Can you work these out from the model? Positions are in its coordinate system, mm. A direction names the side the tool comes from. Give positions to 0.01 mm unless a question says otherwise; leave off trailing zeros. Order: outer loops, then holes, each group sorted by start corner. A loop starts at its lowest first (then second) coordinate and runs counter-clockwise, first axis right, second up. Notation, with made-up numbers: (51, 50.5) -> (91, 50.5) arc R25 ccw to (91, 88.5) -> close; hole circle Ø10 at (-10, 45.5). An arc over 180 degrees is marked (long way). Answer as CSV lines item,"result".
```python
from build123d import *

# Parameters (mm, degrees)
F1_DEPTH = 0.635
F4_DEPTH = 25.4
F2_R     = 3.048
F6_DEPTH = 6.35
F7_DEPTH = 6.35


with BuildPart() as f1:
    # F0 (on Top) → F1 (new body)
    with BuildSketch(Plane.XY):
        with BuildLine():
            Line((0, 0), (89.802561, -89.802561))
            ThreePointArc((89.802561, -89.802561), (127, 0), (89.802561, 89.802561))
            Line((89.802561, 89.802561), (0, 0))
        make_face()
    extrude(amount=F1_DEPTH)

    # F3 (on face) → F4 (intersect)
    with BuildSketch(Plane.XY.offset(0.635)):
        with BuildLine():
            ThreePointArc((53.881537, 53.881537), (76.2, 0), (53.881537, -53.881537))
            Line((53.881537, -53.881537), (89.802561, -89.802561))
            ThreePointArc((89.802561, -89.802561), (127, 0), (89.802561, 89.802561))
            Line((89.802561, 89.802561), (53.881537, 53.881537))
        make_face()
    extrude(amount=-F4_DEPTH, mode=Mode.INTERSECT)

    # F2 (on face) → F6 (join)
    with BuildSketch(Plane.XY.offset(0.635)):
        with Locations((120.65, 0)):
            Circle(F2_R)
    extrude(amount=F6_DEPTH)

    # F5 (on face) → F7 (join)
    with BuildSketch(Plane.XY.offset(0.635)):
        with BuildLine():
            Line((75.810533, -18.372254), (75.810533, -37.168254))
            ThreePointArc((75.810533, -37.168254), (85.208533, -27.770254), (75.810533, -18.372254))
        make_face()
    extrude(amount=F7_DEPTH)


solid = f1.part
```
Item 1: Imagine slicing it at B-B, the plane y = 0. Please give me the cut outline in (x, z) (3 decimals), then the cut area to 3 significant figures.
Numbers:
outline,"(76.2, 0) -> (127, 0) -> (127, 0.635) -> (123.698, 0.635) -> (123.698, 6.985) -> (117.602, 6.985) -> (117.602, 0.635) -> (76.2, 0.635) -> close"
area,"71.0 mm²"
Item 2: Please list where these lines run through material, in increasing order: line 1 along Z through (x, y) = (117, 27.5) (3 decimals); line 2 along X through (y, z) = (-27.5, 3); line 3 along Y through (x, z) = (122, 5.5).
Numbers:
line 1,"z = 0 to 0.635"
line 2,"x = 75.81 to 85.2"
line 3,"y = -2.73 to 2.73"
Item 3: For faces 5 (the cylindrical face through (123.557, 0.916, 3.766)), 6 (the flat face through (72.1, 72.1, 0.3)), 7 (the flat face through (75.811, -28, 4)), which set-ups out of +Z, -Z, +X, -X, +Y, -Y let a thin tool reach every point of the face, with its end or its side?
Numbers:
face 5,"+Z"
face 6,"+Z, -Z, -X, +Y"
face 7,"+Z, -X, +Y, -Y"
Item 4: We'd pull the mould along Y, two halves only. Please class faces 1 (the cylindrical face through (76.195, 0.838, 0.322)), 2 (the flat face through (71.6, -71.6, 0.3)), 3 (the flat face through (90, 1, 0.635)), 4 (the cylindrical face through (85.206, -27.977, 3.766)): released by +Y, released by -Y, zero draft, split by the parting line, or undercut.
Numbers:
face 1,"undercut"
face 2,"released by -Y"
face 3,"zero draft"
face 4,"split by the parting line"
Item 5: Imagine slicing it at A-A, the plane z = 4.75. Please give me the cut outline in (x, y), then the cut area to 3 significant figures.
Numbers:
outline,"(75.81, -37.17) arc R9.4 ccw to (75.81, -18.37) -> close; circle Ø6.1 at (120.65, 0)"
area,"168 mm²"
Item 6: Imagine slicing it at D-D, the plane x = 106. Please give me the cut outline in (y, z) (3 decimals).
Numbers:
outline,"(-69.95, 0) -> (69.95, 0) -> (69.95, 0.635) -> (-69.95, 0.635) -> close"
Item 7: Imagine slicing it at C-C, the plane x = 120.65. Please give me the cut outline in (y, z) (3 decimals).
Numbers:
outline,"(-39.656, 0) -> (39.656, 0) -> (39.656, 0.635) -> (3.048, 0.635) -> (3.048, 6.985) -> (-3.048, 6.985) -> (-3.048, 0.635) -> (-39.656, 0.635) -> close"
Item 8: For pin 1 (3 mm diameter, centred on y = -27.5, z = 4, fed in from -X); pin 2 (6 mm diameter, centred on x = 101.5, y = 67.5, fed in from +Z) (3 decimals); pin 3 (4 mm diameter, centred on y = -55, z = 4, fed in from +X), each with a flat end and sliding along its axis, tell me the tip position at first contact or that it passes through.
Numbers:
pin 1,"stops at x = 75.81"
pin 2,"stops at z = 0.635"
pin 3,"passes through"
